from build123d import *

# Parameters (mm, degrees)
SKETCH1_W                = 3
SKETCH1_H                = 12
BOSS_EXTRUDE1_DEPTH      = 3
ESQUISSE1_W              = 3
ESQUISSE1_H              = 12
BOSS_EXTRU_1_DEPTH       = 25.7
ESQUISSE2_R              = 1
ENL_V_MAT_EXTRU_1_DEPTH  = 4.5
ENL_V_START              = -4.5
ESQUISSE10_R             = 1
ENL_V_MAT_EXTRU_3_DEPTH  = 4.5
ESQUISSE13_W             = 2
ESQUISSE13_H             = 1.5
ENL_V_MAT_EXTRU_5_DEPTH  = 5
ESQUISSE14_W             = 2
ESQUISSE14_H             = 1.5
ENL_V_MAT_EXTRU_6_DEPTH  = 5
BOSS_EXTRUDE2_DEPTH      = 10
BOSS_EXTRUDE2_DEPTH_BACK = 10
SKETCH2_W                = 20
SKETCH2_H                = 2.745941069


with BuildPart() as part:
    # Sketch1 → Boss-Extrude1 (new body)
    with BuildSketch(Plane(origin=(0, 0, 0), x_dir=(1, 0, 0), z_dir=(0, 1, 0))):
        with Locations((13.5, 0)):
            Rectangle(SKETCH1_W, SKETCH1_H)
    extrude(amount=-BOSS_EXTRUDE1_DEPTH)

    # Esquisse1 → Boss.-Extru.1 (add)
    with BuildSketch(Plane(origin=(0, 0, 0), x_dir=(1, 0, 0), z_dir=(0, 1, 0))):
        with Locations((13.5, 0)):
            Rectangle(ESQUISSE1_W, ESQUISSE1_H)
    extrude(amount=BOSS_EXTRU_1_DEPTH)

    # Esquisse2 → Enlèv. mat.-Extru.1 (cut)
    with BuildSketch(Plane(origin=(0, 25.7, 0), x_dir=(1, 0, 0), z_dir=(0, 1, 0))):
        with Locations(Location((13.5, 4, 0), (0, 0, 270))):
            Circle(ESQUISSE2_R)
        with Locations(Location((13.5, -4, 0), (0, 0, 270))):
            Circle(ESQUISSE2_R)
    extrude(amount=-ENL_V_MAT_EXTRU_1_DEPTH, mode=Mode.SUBTRACT)

    # Esquisse10 → Enlèv. mat.-Extru.3 (cut)
    with BuildSketch(Plane.XZ.offset(3).offset(ENL_V_START)):
        with Locations(Location((13.5, -4, 0), (0, 0, 90))):
            Circle(ESQUISSE10_R)
        with Locations(Location((13.5, 4, 0), (0, 0, 90))):
            Circle(ESQUISSE10_R)
    extrude(amount=ENL_V_MAT_EXTRU_3_DEPTH, mode=Mode.SUBTRACT)

    # Esquisse13 → Enlèv. mat.-Extru.5 (cut)
    with BuildSketch(Plane.ZY.offset(-13.5)):
        with Locations((4, -2.25)):
            Rectangle(ESQUISSE13_W, ESQUISSE13_H)
        with Locations((4, 0.75)):
            Rectangle(ESQUISSE13_W, ESQUISSE13_H)
        with Locations((-4, 0.75)):
            Rectangle(ESQUISSE13_W, ESQUISSE13_H)
        with Locations((-4, -2.25)):
            Rectangle(ESQUISSE13_W, ESQUISSE13_H)
        with Locations((-4, 24.95)):
            Rectangle(ESQUISSE13_W, ESQUISSE13_H)
        with Locations((-4, 21.95)):
            Rectangle(ESQUISSE13_W, ESQUISSE13_H)
        with Locations((4, 21.95)):
            Rectangle(ESQUISSE13_W, ESQUISSE13_H)
        with Locations((4, 24.95)):
            Rectangle(ESQUISSE13_W, ESQUISSE13_H)
    extrude(amount=-ENL_V_MAT_EXTRU_5_DEPTH, mode=Mode.SUBTRACT)

    # Esquisse14 → Enlèv. mat.-Extru.6 (cut)
    with BuildSketch(Plane.ZY.offset(-13.5)):
        with Locations((-4, -0.75)):
            Rectangle(ESQUISSE14_W, ESQUISSE14_H)
        with Locations((4, -0.75)):
            Rectangle(ESQUISSE14_W, ESQUISSE14_H)
        with Locations((4, 23.45)):
            Rectangle(ESQUISSE14_W, ESQUISSE14_H)
        with Locations((-4, 23.45)):
            Rectangle(ESQUISSE14_W, ESQUISSE14_H)
    extrude(amount=ENL_V_MAT_EXTRU_6_DEPTH, mode=Mode.SUBTRACT)

    # Sketch2 → Boss-Extrude2 (add, two sides: drawn at the far end of the back side and taken through both)
    with BuildSketch(Plane(origin=(0, 11.35, 0), x_dir=(1, 0, 0), z_dir=(0, 1, 0)).offset(-BOSS_EXTRUDE2_DEPTH_BACK)):
        with Locations((25, -1.372970535)):
            Rectangle(SKETCH2_W, SKETCH2_H)
        with BuildLine():
            ThreePointArc((35, -2.745941069), (39.206766833, -1.17258084), (41.348589647, 2.775196335))
            Line((41.348589647, 2.775196335), (38.555074141, 2.775196335))
            ThreePointArc((38.555074141, 2.775196335), (37.255009249, 0.775948112), (35, 0))
            Line((35, 0), (35, -2.745941069))
        make_face()
        with BuildLine():
            Line((41.348589647, 2.775196335), (38.555074141, 2.775196335))
            ThreePointArc((38.555074141, 2.775196335), (39.951831894, 4.171954088), (41.348589647, 2.775196335))
        make_face()
    extrude(amount=BOSS_EXTRUDE2_DEPTH + BOSS_EXTRUDE2_DEPTH_BACK)


solid = part.part
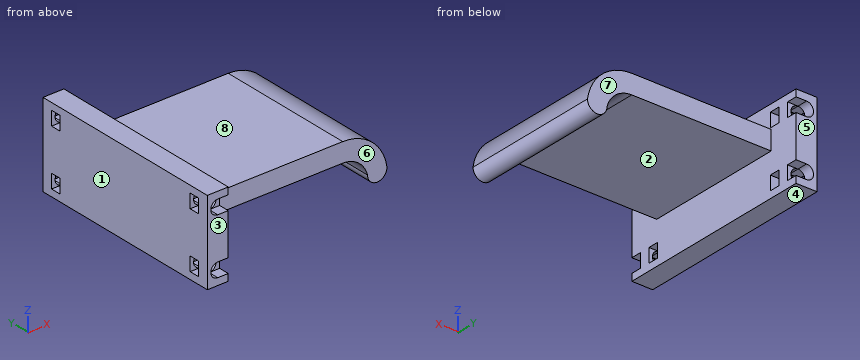
Source: CAD feature listing. Evaluate the final solid. Frame: model axes, mm. Face numbers are marked on the shaded views. A direction names the side the tool comes from. Coordinates: 2 decimals unless noted, no trailing zeros. Order: outer loops, then holes, each group sorted by start corner. A loop starts at its lowest first (then second) coordinate and runs counter-clockwise, first axis right, second up. Notation, with made-up numbers: M 87,79 L 99,79 A15 ccw 99,86 Z; hole C -21,73.25 d6. An arc over 180 degrees is marked long. Write each question's results on one line, items separated by ' | '. Start each with the question number.
Item 1: Cut plane B-B (y = 17.75). Return loops of the section in (x, z).
Item 2: Draft query along X for the marked faces 1, 2 and 3. Return one class per face: pulls with the +X half, pulls with the -X half, needs draft (parallel to the pull), parting line crosses it, or undercut.
Item 3: Cut plane A-A (z = 4). Return loops of the section in (x, y).
Item 4: Cut plane C-C (x = 30.5). Return loops of the section in (y, z), and give its area (3 significant figures).
Item 5: Line query: probe 1 along X at (y, z) = (11.25, -5.5); probe 2 along Z at (x, y) = (22.25, 21); probe 3 along Y at (x, z) = (36.5, 1.5). Output: solid intervals per line, ascending.
Item 6: First-contact query: pin 1 Ø6 at (x, y) = (20, 7) entering from -Z; pin 2 Ø1.5 at (x, y) = (36.5, 1.5) entering from +Z; pin 3 Ø8 at (x, y) = (18, 6) entering from +Z; pin 4 Ø1 at (x, y) = (35.5, 19.5) entering from -Z. Flat tips, straight axial feed; report the tip coordinate or a pass-through.
Item 7: Set-up query: the marked faces 4, 5, 6, 7 and 8. Return all of +Z, -Z, +X, -X, +Y, -Y with unobstructed straight access to the full face (end or side cutting, diameter ignored); none if empty.
Checked values:
1) outline: M 12,-6 L 15,-6 L 15,0 L 35,0 A3.66 cw 38.56,-2.78 A1.4 ccw 41.35,-2.78 A6.41 ccw 35,2.75 L 15,2.75 L 15,6 L 12,6 Z
2) face 1: pulls with the -X half | face 2: undercut | face 3: needs draft
3) outline: M 12,-3 L 12.5,-3 L 12.5,-1.5 L 12,-1.5 Z; M 12,0 L 12.5,0 L 12.5,1.5 L 15,1.5 L 15,21.2 L 12.5,21.2 L 12.5,22.7 L 12,22.7 Z; M 12,24.2 L 12.5,24.2 L 12.5,25.7 L 12,25.7 Z; M 14.5,-1.5 L 15,-1.5 L 15,0 L 14.5,0 Z; M 14.5,22.7 L 15,22.7 L 15,24.2 L 14.5,24.2 Z
4) outline: M 1.35,0 L 21.35,0 L 21.35,2.75 L 1.35,2.75 Z | area: 54.9 mm2
5) probe 1: x = 12 to 15 | probe 2: z = 0 to 2.75 | probe 3: y = 1.35 to 21.35
6) pin 1: stops at z = 0 | pin 2: stops at z = 2.7 | pin 3: stops at z = 6 | pin 4: stops at z = -0.14
7) face 4: -Z, +X, -X, +Y, -Y | face 5: +Z, -Z, +X, -X, +Y | face 6: +Z, -Z, +X, -Y | face 7: +Z, -Z, +X, +Y | face 8: +Z, +X, +Y, -Y
